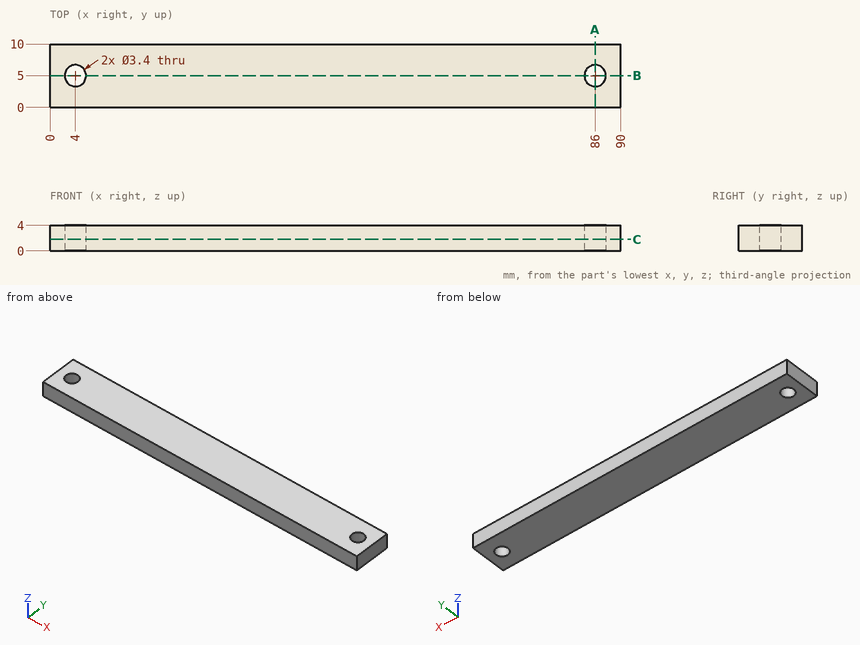
Verification items for this drawing (mm, ordinates from the low corner). Give positions to 0.01 mm unless a question says otherwise; leave off trailing zeros. Loops run counter-clockwise (first coordinate to the right, second up) from the corner with the lowest first, then second, coordinate; pieces in that order, holes last. Notation, with made-up numbers: M -1,4 L 55,4 A9 cw 55,9 Z; hole C 32,71 d4. An arc over 180 degrees is marked long. Answer as a JSON object with one key per item and string values. Group by question number.
Item 1: Sectioned sample at C-C on z = 1.8. Record the boundary of the cut face in (x, y), plus the area to 3 significant figures.
Item 2: Material ranges on L1, parallel to X at y = 5, z = 2.35; L2, parallel to Y at x = 4, z = 1.6; L3, parallel to X at y = 3.75, z = 3.7, recorded low to high.
Item 3: Sectioned sample at A-A on x = 86. Record the boundary of the cut face in (y, z).
Item 4: Sectioned sample at B-B on y = 5. Record the boundary of the cut face in (x, z), plus the area to 3 significant figures.
Findings below:
{
 "1": {"outline": "M 0,0 L 90,0 L 90,10 L 0,10 Z; hole C 4,5 d3.4; hole C 86,5 d3.4", "area": "882 mm2"},
 "2": {"L1": "0 to 2.3, 5.7 to 84.3, 87.7 to 90", "L2": "0 to 3.3, 6.7 to 10", "L3": "0 to 2.85, 5.15 to 84.85, 87.15 to 90"},
 "3": {"outline": "M 0,0 L 3.3,0 L 3.3,4 L 0,4 Z; M 6.7,0 L 10,0 L 10,4 L 6.7,4 Z"},
 "4": {"outline": "M 0,0 L 2.3,0 L 2.3,4 L 0,4 Z; M 5.7,0 L 84.3,0 L 84.3,4 L 5.7,4 Z; M 87.7,0 L 90,0 L 90,4 L 87.7,4 Z", "area": "333 mm2"}
}
